Could you check a few things on this model? Use its own coordinates, in mm. A direction names the side the tool comes from. Give positions to 0.01 mm unless a question says otherwise; leave off trailing zeros. Write each loop counter-clockwise with the first axis right and the second up, starting at its lowest first coordinate (ties: lowest second). Pieces come first, ordered by that corner, then holes. Notation, with made-up numbers: (-10, -2.75) -> (18, -2.75) arc R22 ccw to (18, 24.25) -> close; hole circle Ø5 at (8.25, 72). An arc over 180 degrees is marked (long way). Write item = value, one per line. Start each with the question number.
Autodesk Inventor part; units mm, degrees
ref_plane "Plano de trabajo1" through (0, 5, -50) normal (1, 0, 0) x (0, 0, -1)
ref_plane "Plano de trabajo2" through (0, 15, 0) normal (0, -1, 0) x (1, 0, 0)
ref_plane "YZ Plane" through (0, 0, 0) normal (1, 0, 0) x (0, 1, 0)
sketch "Boceto1" plane through (0, 0, 0) normal (0, 1, 0) x (-1, 0, 0)
  line L0 (27.5, 50) -> (-27.5, 50)
  line L1 (-27.5, 50) -> (-27.5, -50)
  line L2 (-27.5, -50) -> (27.5, -50)
  line L3 (27.5, -50) -> (27.5, 50)
  line L4 (27.5, 50) -> (-27.5, -50) construction
  line L5 (-27.5, 50) -> (27.5, -50) construction
  point P0 (0, 0)
  dimension "d0" = 55
  dimension "d1" = 100
extrude "Extrusión1" add sketch "Boceto1" along normal blind 30
sketch "Boceto2" plane through (27.5, 0, -50) normal (0, 0, -1) x (-1, 0, 0)
  line L0 (22.5, 25) -> (32.5, 25)
  line L1 (32.5, 25) -> (32.5, 5)
  line L2 (32.5, 5) -> (22.5, 5)
  line L3 (22.5, 5) -> (22.5, 25)
  line L4 (22.5, 25) -> (32.5, 5) construction
  line L5 (32.5, 25) -> (22.5, 5) construction
  line L6 (0, 30) -> (55, 30)
  line L7 (0, 0) -> (0, 30)
  line L8 (55, 0) -> (55, 30)
  point P0 (27.5, 0)
  point P1 (27.5, 15)
  point P2 (27.5, 25)
  dimension "d4" = 10
  dimension "d5" = 20
  dimension "d6" = 5
  dimension "d7" = 22.5
  dimension "d24" = 22.5
extrude "Extrusión2" add sketch "Boceto2" along normal blind 10
sketch "Boceto3" plane through (-27.5, 0, 50) normal (0, 0, 1) x (1, 0, 0)
  circle A0 centre (27.5, 20) radius 5
  line L0 (0, 30) -> (55, 30)
  point P0 (27.5, 0)
  point P1 (27.5, 30)
  dimension "d10" = 10
  dimension "d11" = 10
extrude "Extrusión3" cut sketch "Boceto3" against normal blind 15
sketch "Boceto4" plane through (0, 30, 0) normal (0, 1, 0) x (1, 0, 0)
  line L0 (-20, 23) -> (20, 23)
  line L1 (20, 23) -> (20, -23)
  line L2 (20, -23) -> (-20, -23)
  line L3 (-20, -23) -> (-20, 23)
  line L4 (-20, 23) -> (20, -23) construction
  line L5 (20, 23) -> (-20, -23) construction
  point P0 (0, 0)
  dimension "d14" = 40
  dimension "d15" = 46
extrude "Extrusión4" cut sketch "Boceto4" against normal blind 20
ref_plane "Plano de trabajo1" through (0, 5, -50) normal (1, 0, 0) x (0, 0, -1)
sketch "Boceto5" plane through (0, 5, -50) normal (1, 0, 0) x (0, 0, -1)
  line L0 (7.5, 0) -> (0, -2.5)
  line L1 (0, -2.5) -> (0, 0)
  line L2 (0, 0) -> (7.5, 0)
  point P0 (-50, -5)
  point P1 (0, -5)
  point P2 (10, 0)
  dimension "d25" = 2.5
  dimension "d26" = 2.5
extrude "Extrusión5" add sketch "Boceto5" along normal mid plane 8
ref_plane "Plano de trabajo2" through (0, 15, 0) normal (0, -1, 0) x (1, 0, 0)
sketch "Boceto6" plane through (0, 15, 0) normal (0, -1, 0) x (1, 0, 0)
  line L0 (5, -50) -> (8, -50)
  line L1 (27.5, -50) -> (-27.5, -50)
  line L2 (5, -57) -> (8, -50)
  line L3 (4, -50) -> (5, -50)
  line L4 (5, -50) -> (5, -57)
  line L5 (0, -50.2371) -> (0, -56.5746)
  line L6 (-5, -50) -> (-8, -50)
  line L7 (-27.5, -50) -> (27.5, -50)
  line L8 (-5, -57) -> (-8, -50)
  line L9 (-4, -50) -> (-5, -50)
  line L10 (-5, -50) -> (-5, -57)
  point P0 (0, 0)
  point P1 (5, -60)
  point P2 (-5, -60)
  dimension "d29" = 3
  dimension "d30" = 3
extrude "Extrusión6" add sketch "Boceto6" along normal mid plane 8
sketch "Boceto7" plane through (27.5, 0, 50) normal (1, 0, 0) x (0, 0, -1)
  point P0 (50, 0)
ref_plane "Plano de trabajo4" through (-20, 30, -23) normal (0, 0, 1) x (1, 0, 0)
sketch "Boceto8" plane through (27.5, 0, 50) normal (1, 0, 0) x (0, 0, -1)
  line L0 (58, 22) -> (88, 22)
  circle A0 centre (83, 17) radius 1.75
  line L1 (63, 17) -> (83, 17)
  line L2 (88, 22) -> (88, 12)
  circle A1 centre (63, 17) radius 1.75
  line L3 (58, 12) -> (88, 22) construction
  line L4 (58, 22) -> (88, 12) construction
  line L5 (58, 12) -> (58, 22)
  line L6 (88, 12) -> (58, 12)
  line L7 (73, 30) -> (73, 10)
  line L8 (0, 30) -> (100, 30)
  point P0 (50, 0)
  point P1 (72.9522, 12.5553)
  point P2 (57.9522, 14.5161)
  point P3 (72.9522, 12.5553)
  point P4 (88, 17)
  dimension "d34" = 10
  dimension "d35" = 30
  dimension "d36" = 5
  dimension "d37" = 5
  dimension "d38" = 5
  dimension "d39" = 5
  dimension "d40" = 10
  dimension "d41" = 8
hole "Agujero1" at (27.5, 17, -13) at (27.5, 17, -33) direction (-1, 0, 0) diameter 3.5 end through all
split "Dividir1" plane through (-20, 30, -23) removes the side toward (0, 0, -1)
properties part number "camera_support_2_2"
(1) I'm going to push flat-ended pins straight in: pin 1 (5 mm diameter, centred on x = 13.5, z = -4, fed in from +Y); pin 2 (6 mm diameter, centred on x = -4.5, y = 19.5, fed in from -Z). Where does each tip first touch, or does it pass through?
(2) Imagine slicing it at A-A (z = -13). Please give me the cut outline in (x, y), then the cut area to 4 significant figures.
(3) Imagine slicing it at B-B (y = 17). Please give me the cut outline in (x, z), then the cut area to 3 significant figures.
(4) Imagine slicing it at C-C (x = -4). Please give me the cut outline in (y, z).
(5) Imagine slicing it at D-D (z = 7.5). Please give me the cut outline in (x, y).
(6) On a 3-axis mill with a long thin cutter (end or side, diameter ignored), from which of +Z, -Z, +X, -X, +Y, -Y can I reach the whole of each face in a straight line? I mean faces 1 (the flat face through (0, 20, 35)), 2 (the flat face through (-0.4, 14.8, 50)), 3 (the flat face through (-20, 20, 0)). Say none if no direction works.
(7) If I drill on line 1 along X through (y, z) = (27.5, 15); line 2 along Z through (x, y) = (-24.25, 17); line 3 along Y through (x, z) = (0, 42), over which ranges is the centre line in solid material (lowest first)? Write a range as from..to.
(8) We'd pull the mould along Y, two halves only. Please class faces 4 (the cylindrical face through (-23.803, 15.265, -12.772)), 5 (the flat face through (0, 30, 30)), 6 (the flat face through (20, 20, 0)): released by +Y, released by -Y, zero draft, split by the parting line, or undercut.
Answers below:
q1.pin_1 = 10
q1.pin_2 = 23
q2.outline = (-27.5, 0) -> (27.5, 0) -> (27.5, 15.25) -> (20, 15.25) -> (20, 10) -> (-20, 10) -> (-20, 15.25) -> (-27.5, 15.25) -> close; (-27.5, 18.75) -> (-20, 18.75) -> (-20, 30) -> (-27.5, 30) -> close; (20, 18.75) -> (27.5, 18.75) -> (27.5, 30) -> (20, 30) -> close
q2.area = 797.5 mm^2
q3.outline = (-27.5, -23) -> (-20, -23) -> (-20, -14.75) -> (-27.5, -14.75) -> close; (-27.5, -11.25) -> (-20, -11.25) -> (-20, 23) -> (20, 23) -> (20, -11.25) -> (27.5, -11.25) -> (27.5, 50) -> (4, 50) -> (4, 35) -> (-4, 35) -> (-4, 50) -> (-27.5, 50) -> close; (20, -23) -> (27.5, -23) -> (27.5, -14.75) -> (20, -14.75) -> close
q3.area = 2,000 mm^2
q4.outline = (0, -23) -> (10, -23) -> (10, 23) -> (30, 23) -> (30, 50) -> (23, 50) -> (23, 35) -> (17, 35) -> (17, 50) -> (0, 50) -> close
q5.outline = (-27.5, 0) -> (27.5, 0) -> (27.5, 30) -> (20, 30) -> (20, 10) -> (-20, 10) -> (-20, 30) -> (-27.5, 30) -> close
q6.face_1 = +Z
q6.face_2 = +Z, +X, -X, +Y, -Y
q6.face_3 = -Z, +Y
q7.line_1 = -27.5..-20, 20..27.5
q7.line_2 = -23..-14.75, -11.25..50
q7.line_3 = 0..15, 25..30
q8.face_4 = undercut
q8.face_5 = released by +Y
q8.face_6 = zero draft
